Verification items for this drawing (mm, ordinates from the low corner). A direction names the side the tool comes from. Give positions to 0.01 mm unless a question says otherwise; leave off trailing zeros. Loops run counter-clockwise (first coordinate to the right, second up) from the corner with the lowest first, then second, coordinate; pieces in that order, holes last. Notation, with made-up numbers: M 76.25,52 L 103.25,52 A19 ccw 103.25,68 Z; hole C -27.5,24 d5. An arc over 180 degrees is marked long. Answer in a Markdown table with one row per item.
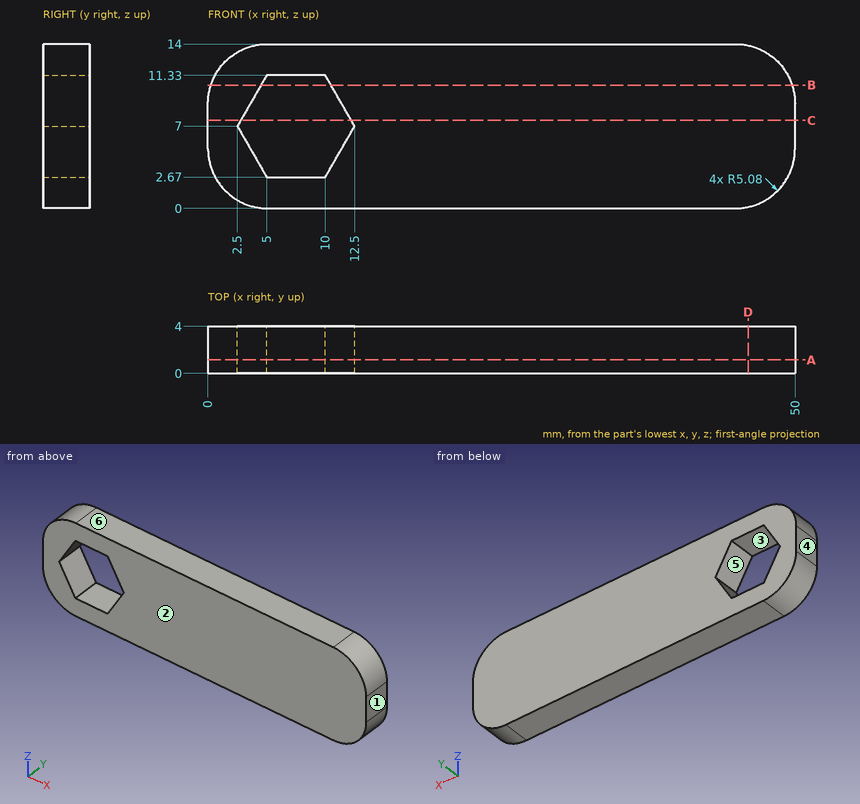
Item 1: Tool access check on the marked faces 5 and 6. Record the directions out of +Z, -Z, +X, -X, +Y, -Y that give a thin tool (end or side, any length) a straight path to the whole face; none if there is none.
Reported:
| item | result |
|---|---|
| face 5 | +Y, -Y |
| face 6 | +Z, +X, -X, +Y, -Y |
Item 2: Release check for a two-part mould opening along X. For the marked faces 1, 2, 3 and 4 record: released by +X, released by -X, zero draft, split by the parting line, or undercut.
Reported:
| item | result |
|---|---|
| face 1 | released by +X |
| face 2 | zero draft |
| face 3 | undercut |
| face 4 | released by -X |
Item 3: Sectioned sample at A-A (y = 1.15). Record the cut outline in (x, z).
Reported:
| item | result |
|---|---|
| outline | M 0,5.08 A5.08 ccw 5.08,0 L 44.92,0 A5.08 ccw 50,5.08 L 50,8.92 A5.08 ccw 44.92,14 L 5.08,14 A5.08 ccw 0,8.92 Z; hole M 2.5,7 L 5,2.67 L 10,2.67 L 12.5,7 L 10,11.33 L 5,11.33 Z |
Item 4: Scan lines: L1, parallel to Z at x = 7, y = 0.4; L2, parallel to X at y = 1.85, z = 11 (1 decimal); L3, parallel to X at y = 3.05, z = 8.5. Record each from-to range of solid material in increasing order. Write a range as [from, to].
Reported:
| item | result |
|---|---|
| L1 | z = [0, 2.67], [11.33, 14] |
| L2 | x = [0.4, 4.8], [10.2, 49.6] |
| L3 | x = [0, 3.37], [11.63, 50] |
Item 5: Go/stop test with flat-tipped pins: pin 1 (1 mm diameter, centred on y = 1, z = 10.5, fed in from -X); pin 2 (1.5 mm diameter, centred on y = 3, z = 2, fed in from +X). Record where each tip stops, or that it passes through.
Reported:
| item | result |
|---|---|
| pin 1 | stops at x = 0.12 |
| pin 2 | stops at x = 49.43 |
Item 6: Sectioned sample at C-C (z = 7.5). Record the cut outline in (x, y), and give its area (3 significant figures).
Reported:
| item | result |
|---|---|
| outline | M 0,0 L 2.79,0 L 2.79,4 L 0,4 Z; M 12.21,0 L 50,0 L 50,4 L 12.21,4 Z |
| area | 162 mm^2 |
Item 7: Sectioned sample at B-B (z = 10.5). Record the cut outline in (x, y).
Reported:
| item | result |
|---|---|
| outline | M 0.25,0 L 4.52,0 L 4.52,4 L 0.25,4 Z; M 10.48,0 L 49.75,0 L 49.75,4 L 10.48,4 Z |
Item 8: Sectioned sample at D-D (x = 46). Record the cut outline in (y, z), and give its area (3 significant figures).
Reported:
| item | result |
|---|---|
| outline | M 0,0.12 L 4,0.12 L 4,13.88 L 0,13.88 Z |
| area | 55.1 mm^2 |
